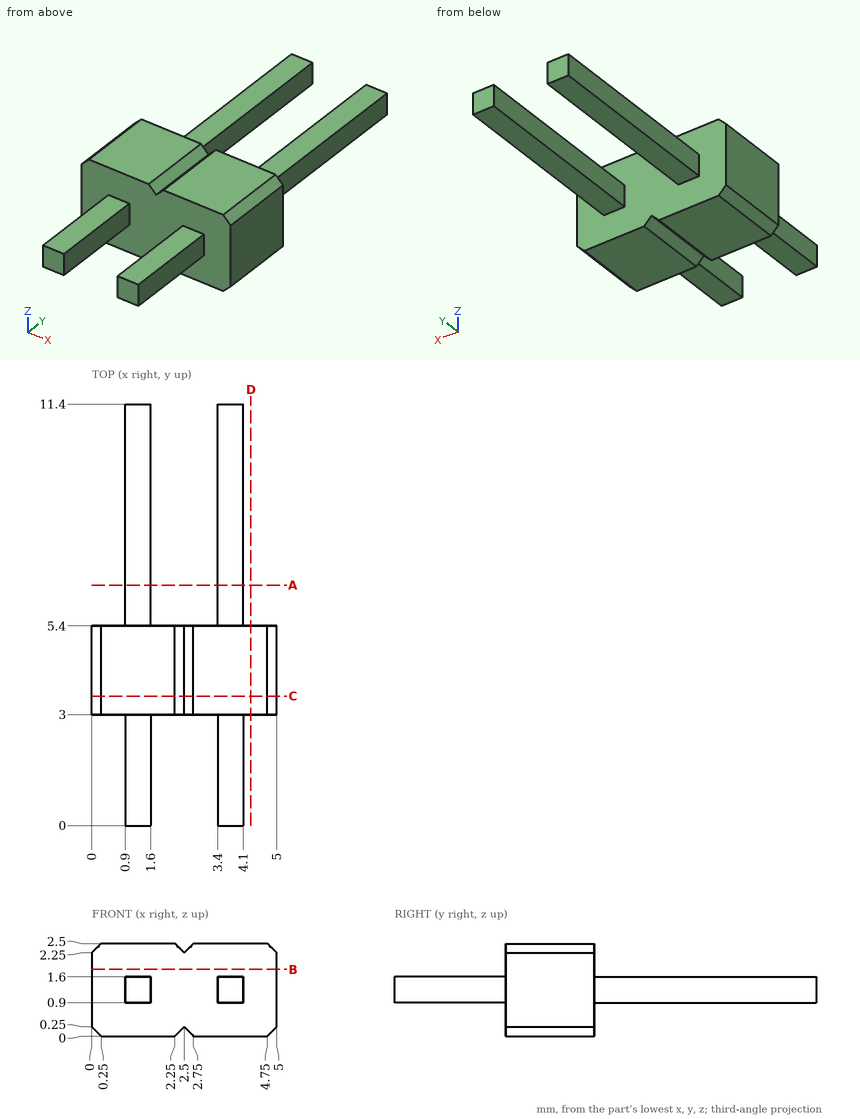
Answer from the drawing. Dimensions are ordinates in mm from the lowest x, y and z of the part. Give positions to 0.01 mm unless a question says otherwise; leave off trailing zeros. Order: outer loops, then holes, each group sorted by start corner. A loop starts at its lowest first (then second) coordinate and runs counter-clockwise, first axis right, second up.
(1) Find section C-C (y = 3.5). Give the vertices of the cut face in (x, z), plus the area to 4 significant figures.
(2) Find section A-A (y = 6.5). Give the vertices of the cut face in (x, z).
(3) Given pin 1 (0.6 mm diameter, centred on y = 1, z = 1, fed in from +X); pin 2 (0.8 mm diameter, centred on y = 9.5, z = 1.5, fed in from -X); pin 3 (1 mm diameter, centred on x = 2, y = 7.5, fed in from +Z), each flat-ended and moving along its own axis, determine where each tip first touches the part or whether it passes through.
(4) Find section D-D (x = 4.3). Give the vertices of the cut face in (y, z), plus the area to 3 significant figures.
(5) Straight lines are drawn through the part: L1, parallel to Y at x = 3.5, z = 2.1; L2, parallel to Z at x = 1, y = 6.5. For each, find the intervals that lie inside material, in ascending order.
(6) Find section B-B (z = 1.8). Give the vertices of the cut face in (x, y), plus the area to 3 significant figures.
Result sheet:
1. outline: (0, 0.25) - (0.25, 0) - (2.25, 0) - (2.5, 0.25) - (2.75, 0) - (4.75, 0) - (5, 0.25) - (5, 2.25) - (4.75, 2.5) - (2.75, 2.5) - (2.5, 2.25) - (2.25, 2.5) - (0.25, 2.5) - (0, 2.25) - close
1. area: 12.25 mm2
2. outline: (0.9, 0.9) - (1.6, 0.9) - (1.6, 1.6) - (0.9, 1.6) - close; (3.4, 0.9) - (4.1, 0.9) - (4.1, 1.6) - (3.4, 1.6) - close
3. pin 1: stops at x = 4.1
3. pin 2: stops at x = 0.9
3. pin 3: stops at z = 1.6
4. outline: (3, 0) - (5.4, 0) - (5.4, 2.5) - (3, 2.5) - close
4. area: 6.00 mm2
5. L1: y = 3 to 5.4
5. L2: z = 0.9 to 1.6
6. outline: (0, 3) - (5, 3) - (5, 5.4) - (0, 5.4) - close
6. area: 12.0 mm2
